Input: part model. Units: mm. Frame: model coordinates. Coordinates: 2 decimals unless noted, no trailing zeros. Write each loop counter-clockwise with the first axis right and the second up, starting at its lowest first coordinate (ties: lowest second). Pieces come first, ordered by that corner, then holes. Notation, with made-up numbers: (67, -31) -> (80, -31) arc R26 ccw to (80, -7) -> close; hole circle Ø2 at (53, -11). An arc over 180 degrees is marked (long way). Use one line per item in the form item = value. Start each with the question number.
(1) First-contact query: pin 1 (1.8 mm diameter, centred on y = -238, z = 3.5, fed in from +X); pin 2 (3 mm diameter, centred on y = -162.5, z = 2, fed in from -X); pin 3 (3 mm diameter, centred on x = -303.5, z = 3.5, fed in from -Y). Flat tips, straight axial feed; report the tip coordinate or a pass-through.
(2) Cut plane B-B on y = -212. Return the cut outline in (x, z), plus the area to 3 significant figures.
(3) Cut plane A-A on z = 4.05. State how many separate pieces and enclosed holes the cut face has, plus the area to 3 significant figures.
(4) Ray query, line 1 along Y through (x, z) = (-246, 3.05); line 2 along X through (y, z) = (69, 5.6). Return the intervals inside material, ascending.
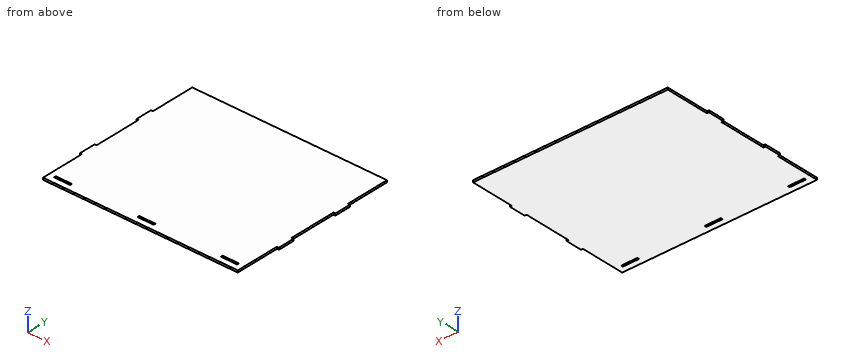
```python
from build123d import *

# Parameters (mm, degrees)
SKETCH1_W           = 50
SKETCH1_H           = 6
BOSS_EXTRUDE1_DEPTH = 6


with BuildPart() as part:
    # Sketch1 → Boss-Extrude1 (new body)
    with BuildSketch(Plane.XY):
        Polygon((-300, 259), (300, 259), (300, 123), (306, 123), (306, 73), (300, 73), (300, -73), (306, -73), (306, -123), (300, -123), (300, -259), (-300, -259), (-300, -123), (-306, -123), (-306, -73), (-300, -73), (-300, 73), (-306, 73), (-306, 123), (-300, 123), align=None)
        with Locations((257, -238)):
            Rectangle(SKETCH1_W, SKETCH1_H, mode=Mode.SUBTRACT)
        with Locations((-257, -238)):
            Rectangle(SKETCH1_W, SKETCH1_H, mode=Mode.SUBTRACT)
        with Locations((0, -238)):
            Rectangle(SKETCH1_W, SKETCH1_H, mode=Mode.SUBTRACT)
    extrude(amount=BOSS_EXTRUDE1_DEPTH)


solid = part.part
```
Values:
q1.pin_1 = 300
q1.pin_2 = -300
q1.pin_3 = -123
q2.outline = (-300, 0) -> (300, 0) -> (300, 6) -> (-300, 6) -> close
q2.area = 3,600 mm2
q3.separate_pieces = 1
q3.enclosed_holes = 3
q3.area = 311,000 mm2
q4.line_1 = -259 to -241, -235 to 259
q4.line_2 = -300 to 300
